from build123d import *

# Parameters (mm, degrees)
F0_W     = 300
F0_H     = 85
F1_DEPTH = 41
F3_W     = 2
F3_H     = 13
F4_DEPTH = 38
F2_W     = 2
F2_H     = 13
F5_DEPTH = 30
F6_R     = 5
F7_R     = 5
F9_DEPTH = 5


with BuildPart() as f1:
    # F0 (on Top) → F1 (new body)
    with BuildSketch(Plane.XY):
        Rectangle(F0_W, F0_H)
    extrude(amount=F1_DEPTH)

    # F3 (on face) → F4 (join)
    with BuildSketch(Plane(origin=(-150, 0, 0), x_dir=(0, -1, 0), z_dir=(-1, 0, 0))):
        with Locations((-20, 11.4)):
            Rectangle(F3_W, F3_H)
    extrude(amount=F4_DEPTH)

    # F2 (on face) → F5 (join)
    with BuildSketch(Plane(origin=(-150, 0, 0), x_dir=(0, -1, 0), z_dir=(-1, 0, 0))):
        with Locations((-35, 19.4)):
            Rectangle(F2_W, F2_H)
    extrude(amount=F5_DEPTH)

    # F6
    f6_edges = [f1.edges().sort_by_distance(p)[0] for p in [
        (-180, 35, 25.9),
        (-180, 35, 12.9),
    ]]
    fillet(f6_edges, radius=F6_R)

    # F7
    f7_edges = [f1.edges().sort_by_distance(p)[0] for p in [
        (-188, 20, 17.9),
        (-188, 20, 4.9),
    ]]
    fillet(f7_edges, radius=F7_R)

    # F8 (on face) → F9 (cut)
    with BuildSketch(Plane.XY.offset(41)):
        Polygon((-62.218837, -15.168179), (41.771069, -15.168179), (41.771069, -32.973677), (109.962918, 0), (41.771069, 33.099085), (41.771069, 15.168179), (-62.218837, 15.168179), align=None)
    extrude(amount=-F9_DEPTH, mode=Mode.SUBTRACT)


solid = f1.part
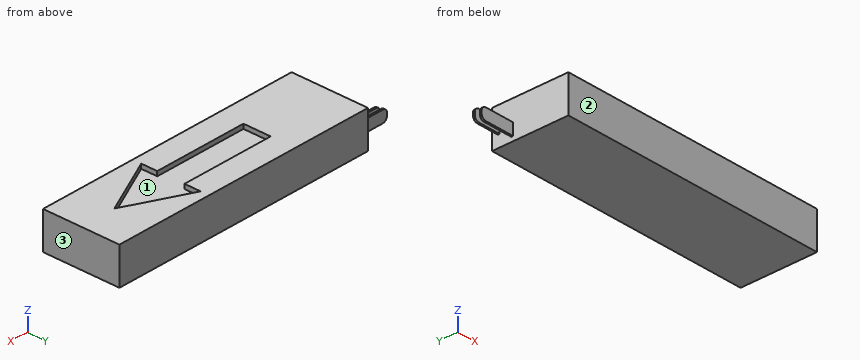
Check sheet for the modelled part. Datum: model origin and axes. Units: mm. Face numbers are marked on the shaded views. Round coordinates to 2 decimals unless told otherwise and drop trailing zeros. Loops run counter-clockwise (first coordinate to the right, second up) from the corner with the lowest first, then second, coordinate; pieces in that order, holes last.
1. Mould release check, pull along X, two halves, no side actions. Record for the marked faces 1, 2 and 3: released by +X, released by -X, zero draft, split by the parting line, or undercut.
2. Scan lines: probe 1 along X at (y, z) = (23, 2); probe 2 along X at (y, z) = (28, 38); probe 3 along Y at (x, z) = (-174, 23). Record each from-to range of solid material in increasing order.
3. Gauge pin test, flat ends, axial feed: pin 1 Ø20.5 at (y, z) = (-2.5, 14.5) entering from -X; pin 2 Ø6.5 at (x, z) = (-162, 14) entering from -Y; pin 3 Ø1.6 at (y, z) = (35.5, 19.5) entering from -X. Record the tip position at first contact, or that the pin passes through.
4. Sectioned sample at A-A on x = -21.5. Record the boundary of the cut face in (y, z).
5. Sectioned sample at C-C on z = 29.5. Record the boundary of the cut face in (x, y).
6. Sectioned sample at B-B on y = 5. Record the boundary of the cut face in (x, z).
Recorded:
1. face 1: undercut
1. face 2: zero draft
1. face 3: released by +X
2. probe 1: x = -150 to 150
2. probe 2: x = -150 to 41.77, 52.28 to 150
2. probe 3: y = 34 to 36
3. pin 1: stops at x = -150
3. pin 2: stops at y = 19
3. pin 3: stops at x = -180
4. outline: (-42.5, 0) - (42.5, 0) - (42.5, 41) - (15.17, 41) - (15.17, 36) - (-15.17, 36) - (-15.17, 41) - (-42.5, 41) - close
5. outline: (-150, -42.5) - (150, -42.5) - (150, 42.5) - (-150, 42.5) - close
6. outline: (-150, 0) - (150, 0) - (150, 41) - (99.66, 41) - (99.66, 36) - (-62.22, 36) - (-62.22, 41) - (-150, 41) - close
